The listing builds one solid part. Answer for the finished solid, in the listing's coordinates (mm). Coordinates: 2 decimals unless noted, no trailing zeros. Write each loop counter-clockwise with the first axis right and the second up, starting at its lowest first coordinate (ties: lowest second). Pieces come first, ordered by that corner, then holes.
from build123d import *

# Parameters (mm, degrees)
SKETCH1_W              = 12.7
SKETCH1_H              = 12.7
BOSS_EXTRUDE1_DEPTH    = 12.7
CUT_EXTRUDE1_DEPTH     = 13.7
F_10_CLEARANCE_HOLE1_D = 5.1054


with BuildPart() as part:
    # Sketch1 → Boss-Extrude1 (new body)
    with BuildSketch(Plane(origin=(0, 0, 0), x_dir=(0, 0, -1), z_dir=(1, 0, 0))):
        with Locations((6.35, 6.35)):
            Rectangle(SKETCH1_W, SKETCH1_H)
    extrude(amount=BOSS_EXTRUDE1_DEPTH)

    # Sketch2 → Cut-Extrude1 (cut, through all)
    with BuildSketch(Plane.XY):
        Polygon((7.332348419, 0), (0, 12.7), (0, 0), align=None)
    extrude(amount=-CUT_EXTRUDE1_DEPTH, mode=Mode.SUBTRACT)

    # #10 Clearance Hole1 (through all)
    with Locations(Plane(origin=(12.7, 6.35, -6.35), x_dir=(0, 0, 1), z_dir=(1, 0, 0))):
        with Locations((0, 0)):
            Hole(F_10_CLEARANCE_HOLE1_D / 2)


solid = part.part
Q1. Find the intervals of material crossed by probe 1 along Y at (x, z) = (11, -6.5); probe 2 along Y at (x, z) = (5, -6.35); probe 3 along Z at (x, y) = (7, 7), in increasing order.
Answers below:
probe 1: y = 0 to 3.8, 8.9 to 12.7
probe 2: y = 8.9 to 12.7
probe 3: z = -12.7 to -8.82, -3.88 to 0
Q2. The part is cut by section C-C, the plane x = 12.25. Write down the section's boundary in (y, z).
Answers below:
outline: (0, -12.7) - (12.7, -12.7) - (12.7, 0) - (0, 0) - close; hole circle Ø5.11 at (6.35, -6.35)
Q3. Determine the mould class of faces 1 (the face through (8.54, 8.842, -5.797)), 2 (the face through (6, 12.7, -6)), 3 (the face through (8, 8, 0)), 4 (the face through (10, 0, -6)) for opening direction Y: released by +Y, released by -Y, zero draft, split by the parting line, or undercut.
Answers below:
face 1: undercut
face 2: released by +Y
face 3: zero draft
face 4: released by -Y
Q4. Given pin 1 (2 mm diameter, centred on x = 9, y = 5, fed in from +Z); pin 2 (3 mm diameter, centred on x = 1.5, z = -3, fed in from -Y); pin 3 (6 mm diameter, centred on y = 6.35, z = -6.35, fed in from -X), each flat-ended and moving along its own axis, determine where each tip first touches the part or whether it passes through.
Answers below:
pin 1: stops at z = 0
pin 2: stops at y = 7.5
pin 3: stops at x = 1.93
Q5. The part is cut by section D-D, the plane z = -1. Write down the section's boundary in (x, y).
Answers below:
outline: (0, 12.7) - (7.33, 0) - (12.7, 0) - (12.7, 12.7) - close
Q6. The part is cut by section B-B, the plane z = -6.5. Write down the section's boundary in (x, y), then the cut area to 3 significant figures.
Answers below:
outline: (0, 12.7) - (2.19, 8.9) - (12.7, 8.9) - (12.7, 12.7) - close; (5.14, 3.8) - (7.33, 0) - (12.7, 0) - (12.7, 3.8) - close
area: 68.7 mm2
Q7. The part is cut by section A-A, the plane y = 6.35. Write down the section's boundary in (x, z).
Answers below:
outline: (3.67, -12.7) - (12.7, -12.7) - (12.7, -8.9) - (3.67, -8.9) - close; (3.67, -3.8) - (12.7, -3.8) - (12.7, 0) - (3.67, 0) - close
